```python
from build123d import *

# Parameters (mm, degrees)
BOSS_EXTRUDE2_DEPTH = 80
SKETCH4_W           = 70
SKETCH4_H           = 250
CUT_EXTRUDE1_DEPTH  = 81
SKETCH5_R           = 20
CUT_EXTRUDE2_DEPTH  = 40


with BuildPart() as part:
    # Sketch1 → Boss-Extrude2 (new body)
    with BuildSketch(Plane(origin=(0, 0, 0), x_dir=(0, 0, -1), z_dir=(1, 0, 0))):
        with BuildLine():
            Line((-20, -150), (-40, -150))
            Line((-40, -150), (-40, 150))
            Line((-40, 150), (40, 150))
            Line((40, 150), (40, -150))
            Line((40, -150), (20, -150))
            ThreePointArc((20, -150), (0, -130), (-20, -150))
        make_face()
    extrude(amount=BOSS_EXTRUDE2_DEPTH)

    # Sketch4 → Cut-Extrude1 (cut, through all)
    with BuildSketch(Plane.XY.offset(40)):
        with Locations((40, -25)):
            Rectangle(SKETCH4_W, SKETCH4_H)
    extrude(amount=-CUT_EXTRUDE1_DEPTH, mode=Mode.SUBTRACT)

    # Sketch5 → Cut-Extrude2 (cut)
    with BuildSketch(Plane(origin=(0, 150, 0), x_dir=(1, 0, 0), z_dir=(0, 1, 0))):
        with Locations((40, 0)):
            Circle(SKETCH5_R)
    extrude(amount=-CUT_EXTRUDE2_DEPTH, mode=Mode.SUBTRACT)


solid = part.part
```
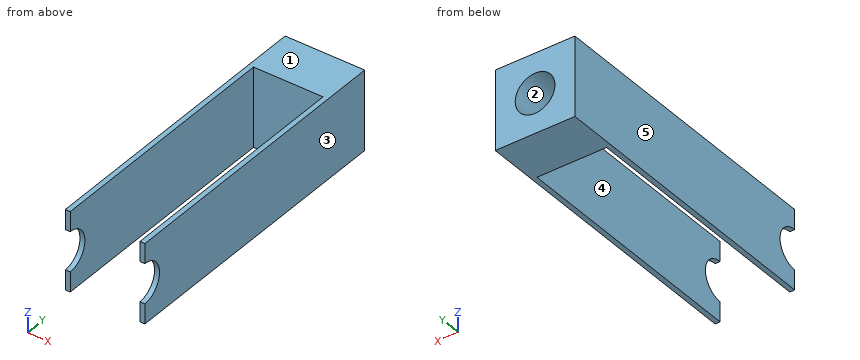
Geometry: final body of the model. Coordinates: model frame, mm. Face numbers are marked on the shaded views. A direction names the side the tool comes from. Coordinates: 2 decimals unless noted, no trailing zeros. Order: outer loops, then holes, each group sorted by start corner. A loop starts at its lowest first (then second) coordinate and runs counter-clockwise, first axis right, second up. Notation, with made-up numbers: (41.25, 39) - (79.25, 39) arc R13 cw to (79.25, 64) - close; hole circle Ø4 at (-31.75, 24.25). An arc over 180 degrees is marked (long way). Return JSON: item names as keys, results as strings. Group by question number.
1. Cut plane C-C (x = 40). Output: boundary loops of the cut face in (y, z), plus the area to 3 significant figures.
2. Pull-direction query (Z, two-part tool) for the marked faces 1, 2 and 3; classes: pulls with the +Z half, pulls with the -Z half, needs draft (parallel to the pull), parting line crosses it, or undercut.
3. Material intervals for line 1 along X through (y, z) = (-55.5, 32); line 2 along Z through (x, y) = (40, 139); line 3 along X through (y, z) = (136, 0), sorted ascending. Write a range as [from, to].
4. Cut plane A-A (y = -2.5). Output: boundary loops of the cut face in (x, z).
5. Cut plane D-D (z = 31.5). Output: boundary loops of the cut face in (x, y), plus the area to 3 significant figures.
6. Cut plane B-B (z = 0). Output: boundary loops of the cut face in (x, y).
7. Set-up query: the marked faces 4 and 5. Return all of +Z, -Z, +X, -X, +Y, -Y with unobstructed straight access to the full face (end or side cutting, diameter ignored); none if empty.
8. Pin query (flat end, axial travel): pin 1 (24 mm diameter, centred on x = 40, z = 0, fed in from +Y); pin 2 (8 mm diameter, centred on x = 42.5, z = -27, fed in from -Y). Return the tip coordinate at first contact, or that it passes through.
Resolved:
{
 "1": {"outline": "(100, -40) - (150, -40) - (150, -20) - (110, -20) - (110, 20) - (150, 20) - (150, 40) - (100, 40) - close", "area": "2,400 mm²"},
 "2": {"face 1": "pulls with the +Z half", "face 2": "undercut", "face 3": "needs draft"},
 "3": {"line 1": "x = [0, 5], [75, 80]", "line 2": "z = [-40, -20], [20, 40]", "line 3": "x = [0, 20], [60, 80]"},
 "4": {"outline": "(0, -40) - (5, -40) - (5, 40) - (0, 40) - close; (75, -40) - (80, -40) - (80, 40) - (75, 40) - close"},
 "5": {"outline": "(0, -150) - (5, -150) - (5, 100) - (75, 100) - (75, -150) - (80, -150) - (80, 150) - (0, 150) - close", "area": "6,500 mm²"},
 "6": {"outline": "(0, -130) - (5, -130) - (5, 100) - (75, 100) - (75, -130) - (80, -130) - (80, 150) - (60, 150) - (60, 110) - (20, 110) - (20, 150) - (0, 150) - close"},
 "7": {"face 4": "+Z, -Z, -Y", "face 5": "+Z, -Z, -X, +Y, -Y"},
 "8": {"pin 1": "stops at y = 110", "pin 2": "stops at y = 100"}
}
